```python
from build123d import *

# Parameters (mm, degrees)
F1_DEPTH = 10
F2_SIZE  = 0.5
F3_SIZE  = 0.2


with BuildPart() as f1:
    # F0 (on Top) → F1 (new body)
    with BuildSketch(Plane.XY):
        Polygon((-51.458716, 10), (-51.458716, 0), (-48.958716, 0), (-48.958716, 2.5), (-47.208716, 2.5), (-47.208716, 0), (-44.708716, 0), (-44.708716, 2.5), (-6.458716, 2.5), (-6.458716, 0), (-3.958716, 0), (-3.958716, 2.5), (-2.208716, 2.5), (-2.208716, 0), (0.291284, 0), (0.291284, 2.5), (38.541284, 2.5), (38.541284, 0), (41.041284, 0), (41.041284, 2.5), (42.791284, 2.5), (42.791284, 0), (45.291284, 0), (45.291284, 10), align=None)
    extrude(amount=F1_DEPTH)

    # F2
    f2_edges = [f1.edges().sort_by_distance(p)[0] for p in [
        (-48.958716, 0, 5),
        (-47.208716, 0, 5),
        (-2.208716, 0, 5),
        (-3.958716, 0, 5),
        (42.791284, 0, 5),
        (41.041284, 0, 5),
    ]]
    chamfer(f2_edges, length=F2_SIZE)

    # F3
    f3_edges = [f1.edges().sort_by_distance(p)[0] for p in [
        (-50.458716, 0, 10),
        (-49.208716, 0.25, 10),
        (-51.458716, 5, 10),
        (-48.958716, 1.5, 10),
        (-3.083716, 10, 10),
        (-48.083716, 2.5, 10),
        (45.291284, 5, 10),
        (-47.208716, 1.5, 10),
        (44.291284, 0, 10),
        (-46.958716, 0.25, 10),
        (43.041284, 0.25, 10),
        (-45.708716, 0, 10),
        (42.791284, 1.5, 10),
        (-44.708716, 1.25, 10),
        (41.916284, 2.5, 10),
        (-25.583716, 2.5, 10),
        (41.041284, 1.5, 10),
        (-6.458716, 1.25, 10),
        (40.791284, 0.25, 10),
        (-5.458716, 0, 10),
        (39.541284, 0, 10),
        (-4.208716, 0.25, 10),
        (38.541284, 1.25, 10),
        (-3.958716, 1.5, 10),
        (19.416284, 2.5, 10),
        (-3.083716, 2.5, 10),
        (0.291284, 1.25, 10),
        (-2.208716, 1.5, 10),
        (-0.708716, 0, 10),
        (-1.958716, 0.25, 10),
        (-50.458716, 0, 0),
        (-49.208716, 0.25, 0),
        (-51.458716, 5, 0),
        (-48.958716, 1.5, 0),
        (-3.083716, 10, 0),
        (-48.083716, 2.5, 0),
        (45.291284, 5, 0),
        (-47.208716, 1.5, 0),
        (44.291284, 0, 0),
        (-46.958716, 0.25, 0),
        (43.041284, 0.25, 0),
        (-45.708716, 0, 0),
        (42.791284, 1.5, 0),
        (-44.708716, 1.25, 0),
        (41.916284, 2.5, 0),
        (-25.583716, 2.5, 0),
        (41.041284, 1.5, 0),
        (-6.458716, 1.25, 0),
        (40.791284, 0.25, 0),
        (-5.458716, 0, 0),
        (39.541284, 0, 0),
        (-4.208716, 0.25, 0),
        (38.541284, 1.25, 0),
        (-3.958716, 1.5, 0),
        (19.416284, 2.5, 0),
        (-3.083716, 2.5, 0),
        (0.291284, 1.25, 0),
        (-2.208716, 1.5, 0),
        (-0.708716, 0, 0),
        (-1.958716, 0.25, 0),
    ]]
    chamfer(f3_edges, length=F3_SIZE)


solid = f1.part
```
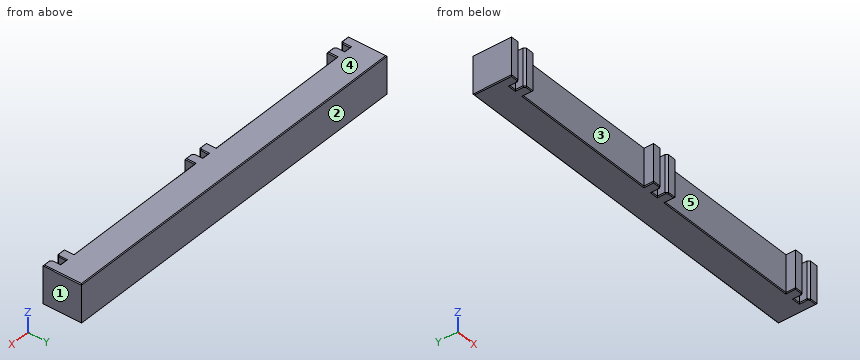
Design review of the part built by this model. Coordinates are the model's own, in mm. Face numbers are marked on the shaded views. A direction names the side the tool comes from. Coordinates: 2 decimals unless noted, no trailing zeros. Order: outer loops, then holes, each group sorted by start corner. A loop starts at its lowest first (then second) coordinate and runs counter-clockwise, first axis right, second up. Notation, with made-up numbers: M 87.5,68.25 L 112.5,68.25 A22 cw 112.5,88.25 Z; hole C 22.25,85 d8. An arc over 180 degrees is marked long. Answer as a JSON object with one key per item and string values. Group by question number.
1) Add section C-C, the plane y = 1.5. Count the separate pieces of the cut face and the enclosed holes in it, then the cut area to 3 significant figures.
2) Mouldability with a two-part tool opening along X and no side actions: class the marked faces 1, 2 and 3 as pulls with the +X half, pulls with the -X half, needs draft (parallel to the pull), parting line crosses it, or undercut.
3) Add section A-A, the plane x = 28.5. Write out the cut boundary in (y, z).
4) For pin 1 (3 mm diameter, centred on x = 13, z = 6, fed in from -Y); pin 2 (1.4 mm diameter, centred on x = 42.5, z = 6, fed in from -Y), all flat-tipped, find the tip position at first contact; note any pin that passes through.
5) Wall thickness on L1, parallel to Y at x = 2.5, z = 3.5: over which ranges is the line inside the solid? List them lowest first.
6) Tool access review of the marked faces 4 and 5: name each direction out of +Z, -Z, +X, -X, +Y, -Y from which nothing blocks a thin tool from reaching the whole face with its end or side.
Computed values:
{
 "1": {"separate pieces": "6", "enclosed holes": "0", "area": "150 mm^2"},
 "2": {"face 1": "pulls with the +X half", "face 2": "needs draft", "face 3": "undercut"},
 "3": {"outline": "M 2.5,0.2 L 2.7,0 L 9.8,0 L 10,0.2 L 10,9.8 L 9.8,10 L 2.7,10 L 2.5,9.8 Z"},
 "4": {"pin 1": "stops at y = 2.5", "pin 2": "stops at y = 0.09"},
 "5": {"L1": "y = 2.5 to 10"},
 "6": {"face 4": "+Z, +X, -X, +Y, -Y", "face 5": "+Z, -Z, -Y"}
}
